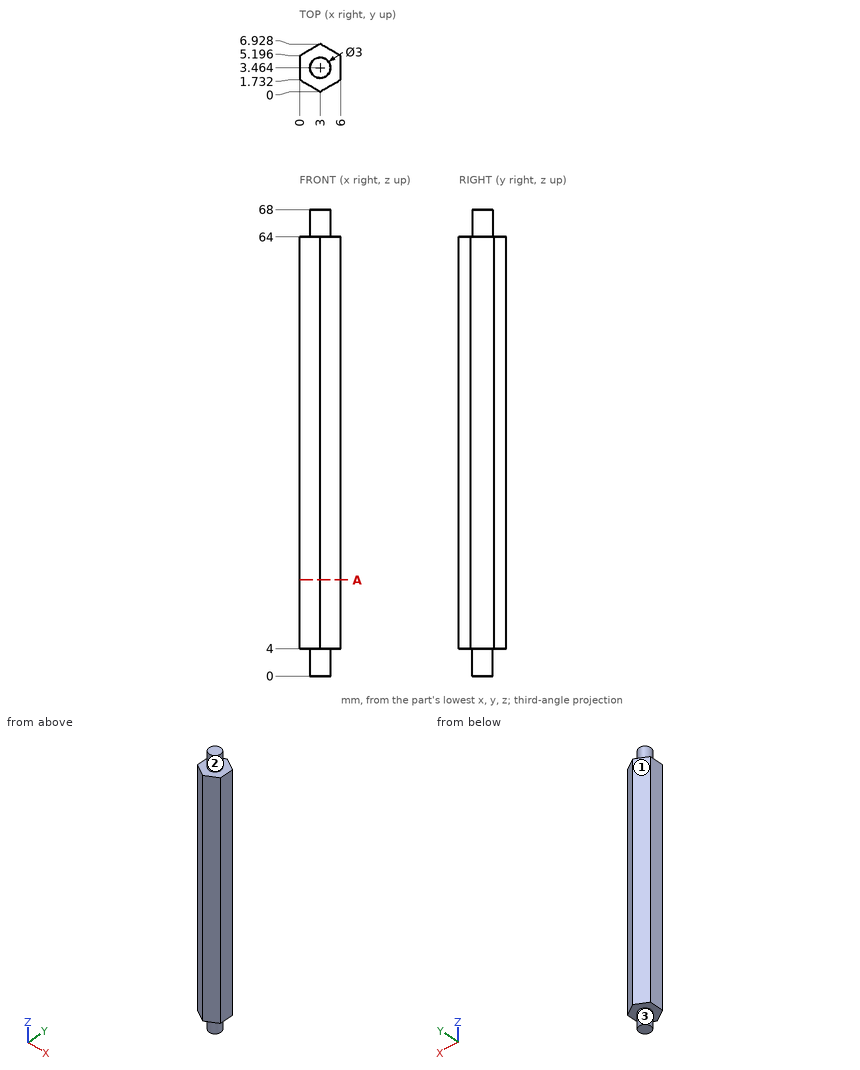
For this review, use the dimensioned drawing (mm, ordinates from the lowest corner) and the shaded views. A direction names the side the tool comes from. Give positions to 0.01 mm unless a question says otherwise; leave off trailing zeros. Loops run counter-clockwise (first coordinate to the right, second up) from the corner with the lowest first, then second, coordinate; pieces in that order, holes last. Notation, with made-up numbers: (-15.75, 14) -> (-8.75, 14) arc R12 ccw to (-8.75, 21) -> close; hole circle Ø9 at (14, 43). An arc over 180 degrees is marked (long way). One line per question, with ' | ' between items. Start each with the question number.
(1) We need section A-A (z = 14). State the section outline as (x, y) points.
(2) For line 1 (Z direction, x = 4.8, y = 2.25); line 2 (Y direction, x = 4.1, z = 58) (1 decimal); line 3 (X direction, y = 6.25, z = 14) (1 decimal), list the stretches that pass through material, from the lowest coordinate up.
(3) Insertion check: P1, Ø1, axis at x = 2, z = 15, coming from the -Y side; P2, Ø1.5, axis at x = 2.5, z = 26, coming from the -Y side; P3, Ø2, axis at x = 1.5, z = 20.5, coming from the +Y side. Each pin has a flat end and moves straight along its axis. Give the tip position at first contact, or say it passes through.
(4) For the marked faces 1, 2 and 3, list the 3-axis set-ups (+Z, -Z, +X, -X, +Y, -Y) from which the entire face can be reached by the end or side of a thin tool; tool diameter is ignored.
The answers:
1) outline: (0, 1.73) -> (3, 0) -> (6, 1.73) -> (6, 5.2) -> (3, 6.93) -> (0, 5.2) -> close
2) line 1: z = 4 to 64 | line 2: y = 0.6 to 6.3 | line 3: x = 1.8 to 4.2
3) P1: stops at y = 0.29 | P2: stops at y = 0 | P3: stops at y = 6.64
4) face 1: +Z, -Z, -X, +Y | face 2: +Z | face 3: -Z
